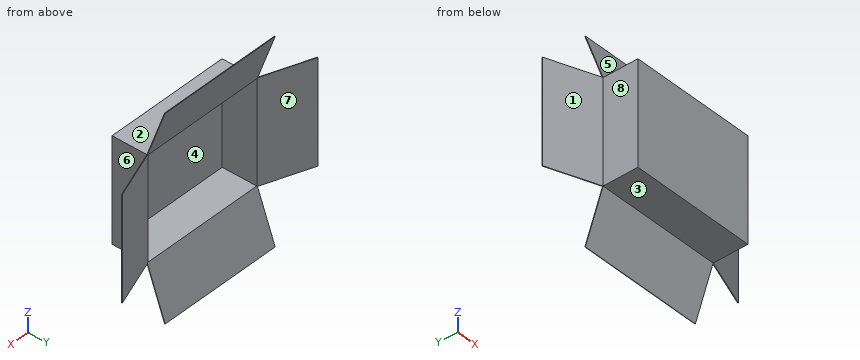
```python
from build123d import *

# Parameters (mm, degrees)
SKETCH1_W           = 423
SKETCH1_H           = 350
BOSS_EXTRUDE1_DEPTH = 119
SHELL1_T            = -2
BOSS_EXTRUDE2_REACH = 474.985
BOSS_EXTRUDE3_REACH = 586.979


with BuildPart() as part:
    # Sketch1 → Boss-Extrude1 (new body)
    with BuildSketch(Plane(origin=(0, 0, 0), x_dir=(1, 0, 0), z_dir=(0, 1, 0))):
        Rectangle(SKETCH1_W, SKETCH1_H)
    extrude(amount=BOSS_EXTRUDE1_DEPTH)

    # Shell1
    shell1_openings = [part.faces().sort_by_distance(p)[0] for p in [
        (0, 119, 0),
    ]]
    offset(amount=SHELL1_T, openings=shell1_openings, kind=Kind.INTERSECTION)

    # Boss-Extrude2: up to this face of the body (flat: up to its plane)
    boss_extrude2_end = Plane(part.part.faces().sort_by_distance((-211.5, 59.5, 0))[0])
    # Sketch2 → Boss-Extrude2 (add, up to the picked face)
    with BuildSketch(Plane(origin=(211.5, 0, 0), x_dir=(0, 0, -1), z_dir=(1, 0, 0)), mode=Mode.PRIVATE) as boss_extrude2_sk1:
        Polygon((-173, 119), (-339.325593879, 179.537565369), (-340.009634166, 177.658180127), (-173.684040287, 117.120614758), align=None)
    boss_extrude2_tool1 = split(extrude(boss_extrude2_sk1.sketch, amount=-BOSS_EXTRUDE2_REACH, mode=Mode.PRIVATE), bisect_by=boss_extrude2_end, keep=Keep.BOTH, mode=Mode.PRIVATE)
    boss_extrude2 = boss_extrude2_tool1.solids().sort_by(Axis((211.5, 148.32909, 256.504817), (-1, 0, 0)))[0]
    add(boss_extrude2)

    # Boss-Extrude3: up to this face of the body (flat: up to its plane)
    boss_extrude3_end = Plane(part.part.faces().sort_by_distance((0, 58.799792462, 175))[0])
    # Sketch4 → Boss-Extrude3 (add, up to the picked face)
    with BuildSketch(Plane(origin=(0, 0, -175), x_dir=(-1, 0, 0), z_dir=(0, 0, -1)), mode=Mode.PRIVATE) as boss_extrude3_sk1:
        Polygon((-209.5, 119), (-375.825593879, 179.537565369), (-376.509634166, 177.658180127), (-210.184040287, 117.120614758), align=None)
    boss_extrude3_tool1 = split(extrude(boss_extrude3_sk1.sketch, amount=-BOSS_EXTRUDE3_REACH, mode=Mode.PRIVATE), bisect_by=boss_extrude3_end, keep=Keep.BOTH, mode=Mode.PRIVATE)
    boss_extrude3 = boss_extrude3_tool1.solids().sort_by(Axis((293.004817, 148.32909, -175), (0, 0, 1)))[0]
    add(boss_extrude3)

    # Mirror1: Boss-Extrude2 across plane
    add(boss_extrude2.mirror(Plane.XY))

    # Mirror2: Boss-Extrude3 across plane
    add(boss_extrude3.mirror(Plane(origin=(0, 0, 0), x_dir=(0, 0, 1), z_dir=(1, 0, 0))))


solid = part.part
```
The model under review builds one solid part; all positions refer to its coordinate system, in mm. Face numbers are marked on the shaded views. A direction names the side the tool comes from. Give positions to 0.01 mm unless a question says otherwise; leave off trailing zeros. Write each loop counter-clockwise with the first axis right and the second up, starting at its lowest first coordinate (ties: lowest second). Pieces come first, ordered by that corner, then holes.
(1) Consider section A-A, the plane y = 37. Give the boundary of the cut face in (x, z).
(2) Consider section B-B, the plane z = 103. Give the boundary of the cut face in (x, y), and give its area (3 significant figures).
(3) For P1, Ø6, axis at x = 95.5, y = 33.5, coming from the -Z side; P2, Ø5, axis at y = 105.5, z = 95, coming from the +X side; P3, Ø4, axis at x = 40, y = 64, coming from the +Z side, all flat-tipped, find the tip position at first contact; note any pin that passes through.
(4) To check wall thickness, follow L1, parallel to X at y = 87, z = 97.5; L2, parallel to Z at x = 159, y = 69; L3, parallel to Y at x = -84, z = -9.5. State the ranges of each line that lie inside material, in increasing order.
(5) Consider section C-C, the plane x = -30.5. Give the boundary of the cut face in (y, z).
(6) Tool access review of the marked faces 1, 2, 3 and 4: name each direction out of +Z, -Z, +X, -X, +Y, -Y from which nothing blocks a thin tool from reaching the whole face with its end or side.
(7) Consider section D-D, the plane z = -266. Give the boundary of the cut face in (x, y).
(8) The part is to be moulded in two halves that separate along X. For the marked faces 5, 6, 7 and 8, say which applies: released by +X, released by -X, zero draft, split by the parting line, or undercut.
Returned:
1. outline: (-211.5, -175) - (211.5, -175) - (211.5, 175) - (-211.5, 175) - close; hole (-209.5, -173) - (209.5, -173) - (209.5, 173) - (-209.5, 173) - close
2. outline: (-376.51, 177.66) - (-211.5, 117.6) - (-211.5, 0) - (211.5, 0) - (211.5, 117.6) - (376.51, 177.66) - (375.83, 179.54) - (209.5, 119) - (209.5, 2) - (-209.5, 2) - (-209.5, 119) - (-375.83, 179.54) - close
2. area: 2,020 mm2
3. P1: stops at z = -175
3. P2: stops at x = 211.5
3. P3: stops at z = 175
4. L1: x = -211.5 to -209.5, 209.5 to 211.5
4. L2: z = -175 to -173, 173 to 175
4. L3: y = 0 to 2
5. outline: (0, -175) - (117.6, -175) - (177.66, -340.01) - (179.54, -339.33) - (119, -173) - (2, -173) - (2, 173) - (119, 173) - (179.54, 339.33) - (177.66, 340.01) - (117.6, 175) - (0, 175) - close
6. face 1: +Z, -Z, -X, -Y
6. face 2: +Z, +X, -X, -Y
6. face 3: -Z, +X, -X, -Y
6. face 4: +Y
7. outline: (-211.5, 150.72) - (211.5, 150.72) - (211.5, 152.85) - (-211.5, 152.85) - close
8. face 5: zero draft
8. face 6: released by +X
8. face 7: undercut
8. face 8: released by -X
